Autodesk Inventor part; units mm, degrees
ref_plane "YZ Plane" through (0, 0, 0) normal (1, 0, 0) x (0, 1, 0)
ref_plane "XZ Plane" through (0, 0, 0) normal (0, 1, 0) x (-1, 0, 0)
ref_plane "XY Plane" through (0, 0, 0) normal (0, 0, 1) x (1, 0, 0)
sketch "Sketch1" plane through (0, 0, 0) normal (0, 1, 0) x (-1, 0, 0)
  circle A0 centre (0, 0) radius 1.5
  dimension "d0" = 3
extrude "Extrusion1" add sketch "Sketch1" along normal blind 12
sketch "Sketch2" plane through (0, 12, 0) normal (0, 1, 0) x (1, 0, 0)
  circle A0 centre (0, 0) radius 1.5
  circle A1 centre (0, 0) radius 2.75
  dimension "d3" = 5.5
extrude "Extrusion2" add sketch "Sketch2" along normal blind 3 contours A0 | A1
sketch "Sketch3" plane through (0, 15, 0) normal (0, 1, 0) x (1, 0, 0)
  circle A0 centre (0, 0) radius 2.75
  line L0 (0, 1.4434) -> (1.25, 0.7217)
  line L1 (1.25, 0.7217) -> (1.25, -0.7217)
  line L2 (1.25, -0.7217) -> (0, -1.4434)
  line L3 (0, -1.4434) -> (-1.25, -0.7217)
  line L4 (-1.25, -0.7217) -> (-1.25, 0.7217)
  line L5 (-1.25, 0.7217) -> (0, 1.4434)
  dimension "d6" = 2.5
extrude "Extrusion3" cut sketch "Sketch3" against normal blind 2 contours L0 L1 L2 L3 L4 L5
thread "Thread1"
chamfer "Chamfer1" distance 0.5 angle 45 1 edges at (1.5, 0, 0)
properties part number "M3x12SHCS"
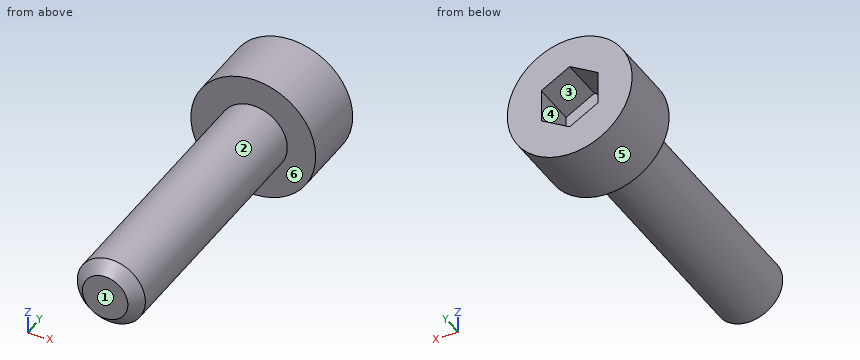
Work out the finished part from the listing and answer in its coordinate system (mm). Face numbers are marked on the shaded views. A direction names the side the tool comes from. Give positions to 0.01 mm unless a question says otherwise; leave off trailing zeros. Order: outer loops, then holes, each group sorted by start corner. A loop starts at its lowest first (then second) coordinate and runs counter-clockwise, first axis right, second up. Notation, with made-up numbers: M 29.25,30.5 L 33.25,30.5 A19 ccw 33.25,59.5 Z; hole C 56.5,-22 d11. An arc over 180 degrees is marked long. Return JSON: item names as keys, results as strings.
1) Section B-B, the plane x = -2.2 is taken. Write down the section's boundary in (y, z).
Resolved:
{"outline": "M 12,-1.65 L 15,-1.65 L 15,1.65 L 12,1.65 Z"}
2) Section C-C, the plane y = 3.75 is taken. Write down the section's boundary in (x, z).
Resolved:
{"outline": "C 0,0 d3"}
3) For a pull along Z with two mould halves and no side action, classify the marked faces 3, 4, 5 and 6 as +Z half, -Z half, draft (parallel to the pull), parting line (faces both ways), or undercut.
Resolved:
{"face 3": "undercut", "face 4": "undercut", "face 5": "parting line", "face 6": "draft"}
4) Straight lines are drawn through the part: line 1 along Y through (x, z) = (-0.3, -0.05); line 2 along Z through (x, y) = (1.2, 13.5); line 3 along Z through (x, y) = (0.05, 13.75). For each, find the intervals that lie inside material, in ascending order. Write a range as [from, to].
Resolved:
{"line 1": "[0, 13]", "line 2": "[-2.47, -0.75], [0.75, 2.47]", "line 3": "[-2.75, -1.41], [1.41, 2.75]"}
5) A tool of negligible diameter and unlimited length cuts with its end or side. For the marked faces 1 and 2, from which of +Z, -Z, +X, -X, +Y, -Y can it reach the whole face along a straight path? Write none if from no direction.
Resolved:
{"face 1": "+Z, -Z, +X, -X, -Y", "face 2": "-Y"}
6) Section A-A, the plane z = 0 is taken. Write down the section's boundary in (x, y), plus the area to 4 significant figures.
Resolved:
{"outline": "M -2.75,12 L -1.5,12 L -1.5,0.5 L -1,0 L 1,0 L 1.5,0.5 L 1.5,12 L 2.75,12 L 2.75,15 L 1.25,15 L 1.25,13 L -1.25,13 L -1.25,15 L -2.75,15 Z", "area": "47.25 mm^2"}
7) Section D-D, the plane z = -1.7 is taken. Write down the section's boundary in (x, y), plus the area to 3 significant figures.
Resolved:
{"outline": "M -2.16,12 L 2.16,12 L 2.16,15 L -2.16,15 Z", "area": "13.0 mm^2"}
8) Each of these flat-tipped pins is pushed along its axis until it touches: pin 1 (3 mm diameter, centred on x = 1.5, y = 2.5, fed in from -Z); pin 2 (2 mm diameter, centred on x = 0, z = 0, fed in from +Y); pin 3 (0.7 mm diameter, centred on y = 14, z = -0.5, fed in from +X). Where does it stop, or does it pass through?
Resolved:
{"pin 1": "z = -1.5", "pin 2": "y = 13", "pin 3": "x = 2.75"}
